For this review, take the finished solid that the model builds, in its own axes (mm). A direction names the side the tool comes from. Coordinates: 2 decimals unless noted, no trailing zeros. Loops run counter-clockwise (first coordinate to the right, second up) from the corner with the lowest first, then second, coordinate; pieces in that order, holes last. Notation, with made-up numbers: M 31.5,-34.75 L 70.5,-34.75 A22 cw 70.5,-16.75 Z; hole C 60.25,42.5 d11. An arc over 180 degrees is marked long. Use one line per item in the form item = value.
```python
from build123d import *

# Parameters (mm, degrees)
SKETCH1_R           = 12.5
BOSS_EXTRUDE1_DEPTH = 11


with BuildPart() as part:
    # Sketch1 → Boss-Extrude1 (new body, symmetric)
    with BuildSketch(Plane.XY):
        with BuildLine():
            Line((-55, 0), (55, 0))
            Line((55, 0), (55, 25))
            Line((55, 25), (28, 25))
            Line((28, 25), (28, 38))
            ThreePointArc((28, 38), (0, 66), (-28, 38))
            Line((-28, 38), (-28, 25))
            Line((-28, 25), (-55, 25))
            Line((-55, 25), (-55, 0))
        make_face()
        with Locations((0, 38)):
            Circle(SKETCH1_R, mode=Mode.SUBTRACT)
    extrude(amount=BOSS_EXTRUDE1_DEPTH, both=True)


solid = part.part
```
1. Consider section C-C on y = 30.5. Write out the cut boundary in (x, z), plus the area to 3 significant figures.
Computed values:
outline = M -28,-11 L -10,-11 L -10,11 L -28,11 Z; M 10,-11 L 28,-11 L 28,11 L 10,11 Z
area = 792 mm2
2. Consider section D-D on x = -47. Write out the cut boundary in (y, z).
Computed values:
outline = M 0,-11 L 25,-11 L 25,11 L 0,11 Z
3. Tool access review of faces 1 (the face through (-41, 25, 0)), 2 (the face through (55, 12, 0)), 3 (the face through (28, 31, 0)): name each direction out of +Z, -Z, +X, -X, +Y, -Y from which nothing blocks a thin tool from reaching the whole face with its end or side.
Computed values:
face_1 = +Z, -Z, -X, +Y
face_2 = +Z, -Z, +X, +Y, -Y
face_3 = +Z, -Z, +X, +Y
4. For pin 1 Ø6.5 at (y, z) = (31.5, -3) entering from +X; pin 2 Ø10.5 at (y, z) = (32.5, 1) entering from -X; pin 3 Ø22.5 at (x, y) = (0, 38) entering from +Z; pin 4 Ø2 at (y, z) = (41.5, -3.5) entering from +X, all flat-tipped, find the tip position at first contact; note any pin that passes through.
Computed values:
pin_1 = 28
pin_2 = -28
pin_3 = through
pin_4 = 27.89
5. Consider section B-B on z = -6.5. Write out the cut boundary in (x, y), plus the area to 3 significant figures.
Computed values:
outline = M -55,0 L 55,0 L 55,25 L 28,25 L 28,38 A28 ccw -28,38 L -28,25 L -55,25 Z; hole C 0,38 d25
area = 4,220 mm2
6. Draft analysis for pull direction Y (two halves, no side actions). For faces 4 (the face through (-2.71, 25.797, -0.154)), 5 (the face through (-28, 32, 0)), 6 (the face through (42, 25, 0)), state which applies: +Y half, -Y half, draft (parallel to the pull), parting line (faces both ways), or undercut.
Computed values:
face_4 = undercut
face_5 = draft
face_6 = +Y half
7. Consider section A-A on x = 0. Write out the cut boundary in (y, z), plus the area to 3 significant figures.
Computed values:
outline = M 0,-11 L 25.5,-11 L 25.5,11 L 0,11 Z; M 50.5,-11 L 66,-11 L 66,11 L 50.5,11 Z
area = 902 mm2
8. Wall thickness on line 1 along Y through (x, z) = (0, 3.25); line 2 along X through (y, z) = (29.5, -0.25); line 3 along Y through (x, z) = (-35, -0.5): over which ranges is each line inside the solid? List them lowest first. Write a range as from..to.
Computed values:
line_1 = 0..25.5, 50.5..66
line_2 = -28..-9.17, 9.17..28
line_3 = 0..25
